```python
from build123d import *

# Parameters (mm, degrees)
SKETCH1_W                 = 45.72
SKETCH1_H                 = 482.6
BOSS_EXTRUDE1_DEPTH       = 45.72
SHELL1_T                  = -2.54
SKETCH5_W                 = 40.64
SKETCH5_H                 = 40.64
CUT_EXTRUDE1_DEPTH        = 2.54
F_97_0_5_DIAMETER_HOLE1_D = 12.7
F_97_0_5_DIAMETER_HOLE2_D = 12.7


with BuildPart() as part:
    # Sketch1 → Boss-Extrude1 (new body)
    with BuildSketch(Plane.XY):
        with Locations((22.86, -241.3)):
            Rectangle(SKETCH1_W, SKETCH1_H)
    extrude(amount=BOSS_EXTRUDE1_DEPTH)

    # Shell1
    shell1_openings = [part.faces().sort_by_distance(p)[0] for p in [
        (22.86, 0, 22.86),
    ]]
    offset(amount=SHELL1_T, openings=shell1_openings, kind=Kind.INTERSECTION)

    # Sketch5 → Cut-Extrude1 (cut)
    with BuildSketch(Plane.XZ.offset(482.6)):
        with Locations((22.86, 22.86)):
            Rectangle(SKETCH5_W, SKETCH5_H)
    extrude(amount=-CUT_EXTRUDE1_DEPTH, mode=Mode.SUBTRACT)

    # #97 (0.5) Diameter Hole1 (through all)
    with Locations(Plane(origin=(22.86, -38.1, 45.72), x_dir=(1, 0, 0), z_dir=(0, 0, 1))):
        with Locations((0, 0), (0, -190.5), (0, -381)):
            Hole(F_97_0_5_DIAMETER_HOLE1_D / 2)

    # #97 (0.5) Diameter Hole2 (through all)
    with Locations(Plane(origin=(45.72, -114.3, 22.86), x_dir=(0, 1, 0), z_dir=(1, 0, 0))):
        with Locations((0, 0), (-50.8, 0), (-101.6, 0), (-152.4, 0), (-203.2, 0), (-254, 0)):
            Hole(F_97_0_5_DIAMETER_HOLE2_D / 2)


solid = part.part
```
Here's how the part is built. I have some questions about the finished solid (model axes, mm). A direction names the side the tool comes from. Coordinates: 2 decimals unless noted, no trailing zeros. Order: outer loops, then holes, each group sorted by start corner. A loop starts at its lowest first (then second) coordinate and runs counter-clockwise, first axis right, second up.
1) Will these pins go through, and if not, where does the flat tip stop? pin 1 (12 mm diameter, centred on x = 14, z = 14, fed in from +Y); pin 2 (20.5 mm diameter, centred on x = 22.86, y = -38.1, fed in from -Z).
2) We'd pull the mould along Y, two halves only. Please class faces 1 (the face through (1.252, -171.157, 24.767)), 2 (the face through (23, -245, 43.18)), 3 (the face through (2, 0, 19)): +Y half, -Y half, draft (parallel to the pull), parting line (faces both ways), or undercut.
3) Imagine slicing it at A-A on z = 39. List the corners of the cut face in (x, y) for me.
4) Imagine slicing it at C-C on x = 22.86. State how many separate pieces and enclosed holes the cut face has, and give its area (3 significant figures).
5) I need wall thicknesses on line 1 (X direction, y = -204, z = 25); line 2 (Z direction, x = 44, y = -317.5). Which ranges of each line are inside material? Lowest first, please.
6) Which directions (+Z, -Z, +X, -X, +Y, -Y) give clear straight access to the entire face, cutting with the end or side of a thin tool? Please do faces 4 (the face through (1.252, -311.156, 23.139)), 5 (the face through (23, -245, 2.54)).
7) Imagine slicing it at B-B on y = -200.5. List the corners of the cut face in (x, z) for me.
8) Imagine slicing it at D-D on y = -419.1. List the corners of the cut face in (x, z) for me, and give its area (3 significant figures).
Response values:
1. pin 1: passes through
1. pin 2: stops at z = 0
2. face 1: undercut
2. face 2: draft
2. face 3: +Y half
3. outline: (0, -482.6) - (2.54, -482.6) - (2.54, 0) - (0, 0) - close; (43.18, -482.6) - (45.72, -482.6) - (45.72, 0) - (43.18, 0) - close
4. separate pieces: 8
4. enclosed holes: 0
4. area: 2,260 mm2
5. line 1: x = 0 to 2.54, 43.18 to 45.72
5. line 2: z = 0 to 16.51, 29.21 to 45.72
6. face 4: +X, -X
6. face 5: +Y, -Y
7. outline: (0, 0) - (45.72, 0) - (45.72, 45.72) - (0, 45.72) - close; hole (2.54, 2.54) - (43.18, 2.54) - (43.18, 43.18) - (2.54, 43.18) - close
8. outline: (0, 0) - (16.51, 0) - (16.51, 2.54) - (2.54, 2.54) - (2.54, 43.18) - (16.51, 43.18) - (16.51, 45.72) - (0, 45.72) - close; (29.21, 0) - (45.72, 0) - (45.72, 45.72) - (29.21, 45.72) - (29.21, 43.18) - (43.18, 43.18) - (43.18, 2.54) - (29.21, 2.54) - close
8. area: 374 mm2
